from build123d import *

# Parameters (mm, degrees)
SKETCH5_R           = 3.96
BOSS_EXTRUDE5_DEPTH = 3
BOSS_EXTRUDE7_DEPTH = 5.6
SKETCH7_R           = 3.175
CUT_EXTRUDE1_DEPTH  = 5
SKETCH8_R           = 3.175
BOSS_EXTRUDE9_DEPTH = 1.4


with BuildPart() as part:
    # Sketch5 → Boss-Extrude5 (new body)
    with BuildSketch(Plane(origin=(0, 0, 0), x_dir=(-1, 0, 0), z_dir=(0, 1, 0))):
        with Locations(Location((0, 0, 0), (0, 0, 90))):
            Circle(SKETCH5_R)
    extrude(amount=BOSS_EXTRUDE5_DEPTH)

    # Sketch6 → Boss-Extrude7 (add)
    with BuildSketch(Plane.XZ.offset(-3)):
        Polygon((-4.572614132, 0), (-2.286307066, -3.96), (2.286307066, -3.96), (4.572614132, 0), (2.286307066, 3.96), (-2.286307066, 3.96), align=None)
    extrude(amount=-BOSS_EXTRUDE7_DEPTH)

    # Sketch7 → Cut-Extrude1 (cut)
    with BuildSketch(Plane.XZ):
        with Locations(Location((0, 0, 0), (0, 0, 270))):
            Circle(SKETCH7_R)
    extrude(amount=-CUT_EXTRUDE1_DEPTH, mode=Mode.SUBTRACT)

    # Sketch8 → Boss-Extrude9 (add)
    with BuildSketch(Plane(origin=(0, 8.6, 0), x_dir=(1, 0, 0), z_dir=(0, 1, 0))):
        with Locations(Location((0, 0, 0), (0, 0, 90))):
            Circle(SKETCH8_R)
    extrude(amount=BOSS_EXTRUDE9_DEPTH)


solid = part.part
Geometry: final body of the model. Coordinates: model frame, mm. A direction names the side the tool comes from. Give positions to 0.01 mm unless a question says otherwise; leave off trailing zeros. Write each loop counter-clockwise with the first axis right and the second up, starting at its lowest first coordinate (ties: lowest second). Pieces come first, ordered by that corner, then holes. Notation, with made-up numbers: (27, 59.5) - (73, 59.5) arc R27 ccw to (73, 88.5) - close; hole circle Ø5 at (61, -9). An arc over 180 degrees is marked (long way). Return JSON: item names as keys, results as strings. Group by question number.
1) Line query: line 1 (X direction, y = 1.75, z = 0) (3 decimals); line 2 (Y direction, x = -2.75, z = 2.5); line 3 (Y direction, x = -2.5, z = 1). Output: solid intervals per line, ascending.
2) Mould query, pull axis X, two halves, no side actions, for faces 4 (the flat face through (-3.41, 5.76, 2.01)), 5 (the flat face through (4.13, 3, 0.01)), 6 (the flat face through (0, 5, 0)). Classes: released by +X, released by -X, zero draft, split by the parting line, or undercut.
3) Section B-B on x = -2.75. Return the cut outline in (y, z), plus the area to 3 significant figures.
4) Set-up query: faces 1 (the cylindrical face through (-3.866, 1.479, -0.858)), 2 (the cylindrical face through (1.93, 9.29, 2.52)), 3 (the flat face through (-2, 3, 3.6)). Return all of +Z, -Z, +X, -X, +Y, -Y with unobstructed straight access to the full face (end or side cutting, diameter ignored); none if empty.
5) Section C-C on z = 1.5. Return the cut outline in (x, y).
6) First-contact query: P1, Ø0.6, axis at x = -1, z = 2.5, coming from the -Y side. Flat tip, straight axial feed; report the tip coordinate or a pass-through.
7) Section D-D on y = 7.5. Return the cut outline in (x, z).
8) Section A-A on y = 4.25. Return the cut outline in (x, z) (3 decimals), plus the area to 3 significant figures.
Filled in:
{
 "1": {"line 1": "x = -3.96 to -3.175, 3.175 to 3.96", "line 2": "y = 0 to 8.6", "line 3": "y = 5 to 10"},
 "2": {"face 4": "released by -X", "face 5": "zero draft", "face 6": "undercut"},
 "3": {"outline": "(0, -2.85) - (3, -2.85) - (3, -3.16) - (8.6, -3.16) - (8.6, -1.59) - (10, -1.59) - (10, 1.59) - (8.6, 1.59) - (8.6, 3.16) - (3, 3.16) - (3, 2.85) - (0, 2.85) - (0, 1.59) - (5, 1.59) - (5, -1.59) - (0, -1.59) - close", "area": "41.0 mm^2"},
 "4": {"face 1": "-Y", "face 2": "+Y", "face 3": "+Z, -X, -Y"},
 "5": {"outline": "(-3.71, 3) - (-3.66, 3) - (-3.66, 0) - (-2.8, 0) - (-2.8, 5) - (2.8, 5) - (2.8, 0) - (3.66, 0) - (3.66, 3) - (3.71, 3) - (3.71, 8.6) - (2.8, 8.6) - (2.8, 10) - (-2.8, 10) - (-2.8, 8.6) - (-3.71, 8.6) - close"},
 "6": {"P1": "stops at y = 5"},
 "7": {"outline": "(-4.57, 0) - (-2.29, -3.96) - (2.29, -3.96) - (4.57, 0) - (2.29, 3.96) - (-2.29, 3.96) - close"},
 "8": {"outline": "(-4.573, 0) - (-2.286, -3.96) - (2.286, -3.96) - (4.573, 0) - (2.286, 3.96) - (-2.286, 3.96) - close; hole circle Ø6.35 at (0, 0)", "area": "22.7 mm^2"}
}
